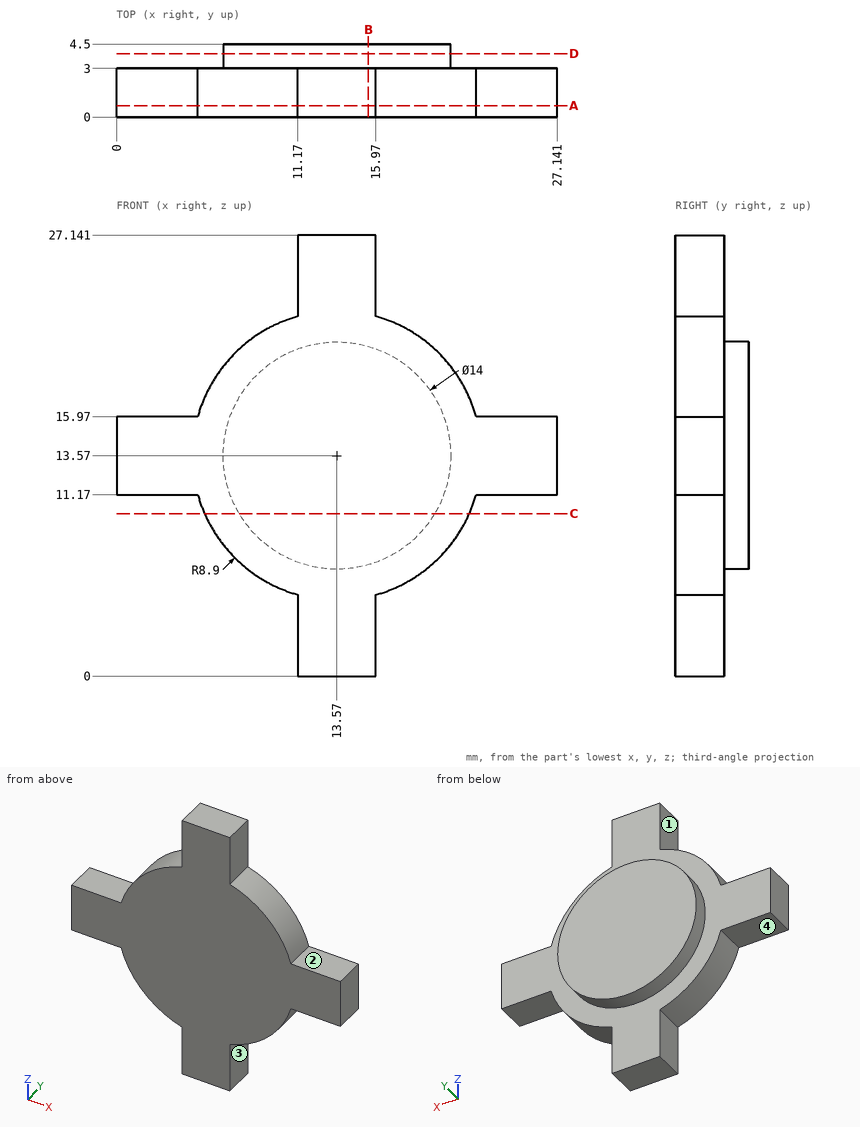
Here's the drawing with two shaded views (mm, measured from the low corner). I have some questions. A direction names the side the tool comes from. Round coordinates to 2 decimals unless told otherwise and drop trailing zeros. Order: outer loops, then holes, each group sorted by start corner. A loop starts at its lowest first (then second) coordinate and runs counter-clockwise, first axis right, second up. Notation, with made-up numbers: (-27.5, 13.5) -> (-3.5, 13.5) arc R21 cw to (-3.5, 26.5) -> close; hole circle Ø5 at (12, -21). An arc over 180 degrees is marked (long way). Use a Markdown table: item, result. Add a question column.
(1) Suppose I cut it at D-D, the plane y = 3.9. Please give me the cut outline in (x, z).
(2) For the marked faces 1, 2, 3 and 4, which set-ups out of +Z, -Z, +X, -X, +Y, -Y let a thin tool reach every point of the face, with its end or its side?
(3) Suppose I cut it at C-C, the plane z = 10. Please give me the cut outline in (x, y).
(4) Suppose I cut it at A-A, the plane y = 0.7. Please give me the cut outline in (x, z).
(5) For pin 1 Ø2.5 at (x, y) = (1.5, 1) entering from -Z; pin 2 Ø2.5 at (y, z) = (1.5, 25.5) entering from +X; pin 3 Ø1.5 at (y, z) = (4, 23.5) entering from +X; pin 4 Ø1.5 at (y, z) = (3, 6) entering from -X, each with a flat end and sliding along its axis, tell me the tip position at first contact or that it passes through.
(6) I need wall thicknesses on line 1 along X through (y, z) = (2.15, 1.75); line 2 along Y through (x, z) = (10.75, 20.5). Which ranges of each line are inside material? Lowest first, please.
(7) Suppose I cut it at B-B, the plane x = 15.5. Please give me the cut outline in (y, z).
Verdict:
| question | item | result |
|---|---|---|
| 1 | outline | circle Ø14 at (13.57, 13.57) |
| 2 | face 1 | +Z, -X, +Y, -Y |
| 2 | face 2 | +Z, +X, +Y, -Y |
| 2 | face 3 | -Z, +X, +Y, -Y |
| 2 | face 4 | -Z, -X, +Y, -Y |
| 3 | outline | (5.42, 0) -> (21.72, 0) -> (21.72, 3) -> (19.59, 3) -> (19.59, 4.5) -> (7.55, 4.5) -> (7.55, 3) -> (5.42, 3) -> close |
| 4 | outline | (0, 11.17) -> (5, 11.17) arc R8.9 ccw to (11.17, 5) -> (11.17, 0) -> (15.97, 0) -> (15.97, 5) arc R8.9 ccw to (22.14, 11.17) -> (27.14, 11.17) -> (27.14, 15.97) -> (22.14, 15.97) arc R8.9 ccw to (15.97, 22.14) -> (15.97, 27.14) -> (11.17, 27.14) -> (11.17, 22.14) arc R8.9 ccw to (5, 15.97) -> (0, 15.97) -> close |
| 5 | pin 1 | z = 11.17 |
| 5 | pin 2 | x = 15.97 |
| 5 | pin 3 | through |
| 5 | pin 4 | x = 7.85 |
| 6 | line 1 | 11.17 to 15.97 |
| 6 | line 2 | 0 to 3 |
| 7 | outline | (0, 0) -> (3, 0) -> (3, 6.84) -> (4.5, 6.84) -> (4.5, 20.3) -> (3, 20.3) -> (3, 27.14) -> (0, 27.14) -> close |
